Read the model definition and answer for the solid it produces. Units are mm, in the model's axes. Round coordinates to 2 decimals unless told otherwise and drop trailing zeros. Write each loop counter-clockwise with the first axis right and the second up, starting at its lowest first coordinate (ties: lowest second). Pieces come first, ordered by that corner, then holes. Notation, with made-up numbers: (50, 57.25) - (59, 57.25) arc R22 ccw to (59, 74.25) - close; hole circle Ø4 at (7, 30.25). An arc over 180 degrees is marked (long way). One line per item, written item: value. Start each with the question number.
(1) Find the intervals of material crossed by L1, parallel to X at y = 0.5, z = 18; L2, parallel to X at y = -7.5, z = 18.5; L3, parallel to Y at x = -0.75, z = 14.25, in increasing order.
(2) The mould has two halves that part along X. Classify faces 1 (the face through (0, 0, 2)), 2 (the face through (0, 0, 0)): +X half, -X half, draft (parallel to the pull), parting line (faces both ways), or undercut.
(3) Flat-ended cylindrical pins translate along their axes: pin 1 Ø4 at (x, y) = (-0.5, 0.5) entering from +Z; pin 2 Ø1 at (y, z) = (7.5, 18) entering from -X; pin 3 Ø5 at (x, z) = (-7.5, 17) entering from -Y. Find the tip coordinate at first contact, or state that the pin passes through.
(4) A cutting plane is placed at A-A, the plane z = 15.5. Determine the outline of the cut face in (x, y), plus the area to 3 significant figures.
(5) A cutting plane is placed at B-B, the plane z = 11. Determine the outline of the cut face in (x, y), plus the area to 3 significant figures.
from build123d import *


with BuildPart() as f1:
    # F0 (on Front) → F1 (revolve)
    with BuildSketch(Plane.XZ):
        with BuildLine():
            Line((0, 2), (0, 0))
            Line((0, 0), (9, 0))
            Line((9, 0), (10.9678164715, 24.5977058939))
            Line((10.9678164715, 24.5977058939), (11, 25))
            Line((11, 25), (8.9936102074, 25))
            Line((8.9936102074, 25), (8.98694515, 24.9166867831))
            Line((8.98694515, 24.9166867831), (7.5217121184, 6.6012738886))
            ThreePointArc((7.5217121184, 6.6012738886), (5.9292702464, 3.3261987971), (2.5376357258, 2))
            Line((2.5376357258, 2), (0, 2))
        make_face()
        with BuildLine():
            Line((8.9936102074, 25), (11, 25))
            ThreePointArc((11, 25), (9.9968051037, 25.8884287672), (8.9936102074, 25))
        make_face()
    revolve(axis=Axis((0, 0, 12.5), (0, 0, 1)))


solid = f1.part
Here are the results:
1. L1: -10.43 to -8.42, 8.42 to 10.43
1. L2: -7.32 to -3.94, 3.94 to 7.32
1. L3: -10.11 to -8.1, 8.1 to 10.11
2. face 1: undercut
2. face 2: draft
3. pin 1: z = 2
3. pin 2: x = -7.75
3. pin 3: y = -9.09
4. outline: circle Ø20.48 at (0, 0); hole circle Ø16.47 at (0, 0)
4. area: 116 mm²
5. outline: circle Ø19.76 at (0, 0); hole circle Ø15.75 at (0, 0)
5. area: 112 mm²
